The listing builds one solid part. Answer for the finished solid, in the listing's coordinates (mm). Round coordinates to 2 decimals unless told otherwise and drop trailing zeros. Order: outer loops, then holes, each group sorted by start corner. A loop starts at its lowest first (then second) coordinate and runs counter-clockwise, first axis right, second up. Notation, with made-up numbers: (74, 6.5) -> (112, 6.5) arc R16 cw to (112, 10.5) -> close; hole circle Ø10 at (74, -28.75). An arc over 180 degrees is marked (long way). Answer in a Markdown table with one row per item. Add a question column.
```python
from build123d import *

# Parameters (mm, degrees)
F0_R     = 100
F1_DEPTH = 25
F2_R     = 10
F3_R     = 4
F4_DEPTH = 25


with BuildPart() as f1:
    # F0 (on Front) → F1 (new body)
    with BuildSketch(Plane.XZ):
        Circle(F0_R)
    extrude(amount=F1_DEPTH)

    # F2
    f2_edges = [f1.edges().sort_by_distance(p)[0] for p in [
        (-100, -25, 0),
    ]]
    fillet(f2_edges, radius=F2_R)

    # F3 (on face) → F4 (cut)
    with BuildSketch(Plane.XZ.offset(25)):
        Circle(F3_R)
    extrude(amount=-F4_DEPTH, mode=Mode.SUBTRACT)


solid = f1.part
```
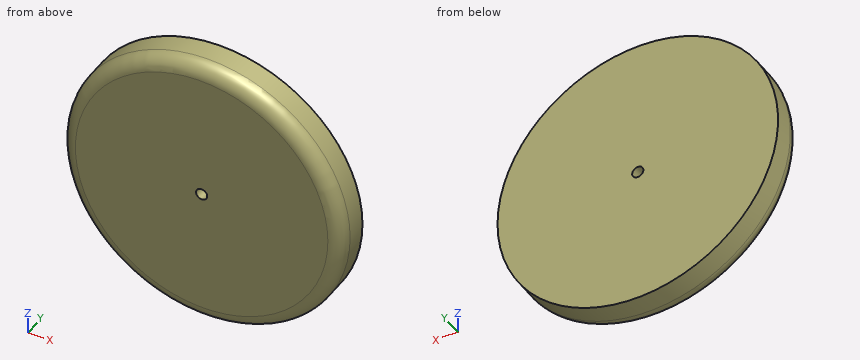
Item 1: The part is cut by section A-A, the plane z = 0. Give the vertices of the cut face in (x, y).
Item 2: Flat-ended cylindrical pins translate along their axes: P1, Ø2, axis at y = -18, z = 37, coming from the -X side; P2, Ø10, axis at x = 40, y = -17, coming from the -Z side; P3, Ø1.5, axis at x = -59.5, y = -10.5, coming from the -Z side. Find the tip coordinate at first contact, or state that the pin passes through.
Item 3: The part is cut by section D-D, the plane y = -22. Give the vertices of the cut face in (x, z), and give its area (3 significant figures).
Item 4: The part is cut by section C-C, the plane y = -2.5. Give the vertices of the cut face in (x, z), and give its area (3 significant figures).
Item 5: The part is cut by section B-B, the plane x = 0. Give the vertices of the cut face in (y, z).
Item 6: Find the intervals of material crossed by probe 1 along Z at (x, y) = (0, -14.5); probe 2 along Z at (x, y) = (-45, -20); probe 3 along Z at (x, y) = (-17, -19), in increasing order. Write a range as [from, to].
Resolved:
| question | item | result |
|---|---|---|
| 1 | outline | (-100, -15) arc R10 ccw to (-90, -25) -> (-4, -25) -> (-4, 0) -> (-100, 0) -> close; (4, -25) -> (90, -25) arc R10 ccw to (100, -15) -> (100, 0) -> (4, 0) -> close |
| 2 | P1 | x = -92.9 |
| 2 | P2 | z = -93.59 |
| 2 | P3 | z = -80.92 |
| 3 | outline | circle Ø194.28 at (0, 0); hole circle Ø8 at (0, 0) |
| 3 | area | 29,600 mm2 |
| 4 | outline | circle Ø200 at (0, 0); hole circle Ø8 at (0, 0) |
| 4 | area | 31,400 mm2 |
| 5 | outline | (-25, -90) arc R10 ccw to (-15, -100) -> (0, -100) -> (0, -4) -> (-25, -4) -> close; (-25, 4) -> (0, 4) -> (0, 100) -> (-15, 100) arc R10 ccw to (-25, 90) -> close |
| 6 | probe 1 | [-100, -4], [4, 100] |
| 6 | probe 2 | [-87.8, 87.8] |
| 6 | probe 3 | [-97.7, 97.7] |
